Design review of the part shown in the three views and the two pictorial views. Dimensions are in mm from the part's minimum x, y and z. Give positions to 0.01 mm unless a question says otherwise; leave off trailing zeros. Order: outer loops, then holes, each group sorted by start corner. A loop starts at its lowest first (then second) coordinate and runs counter-clockwise, first axis right, second up.
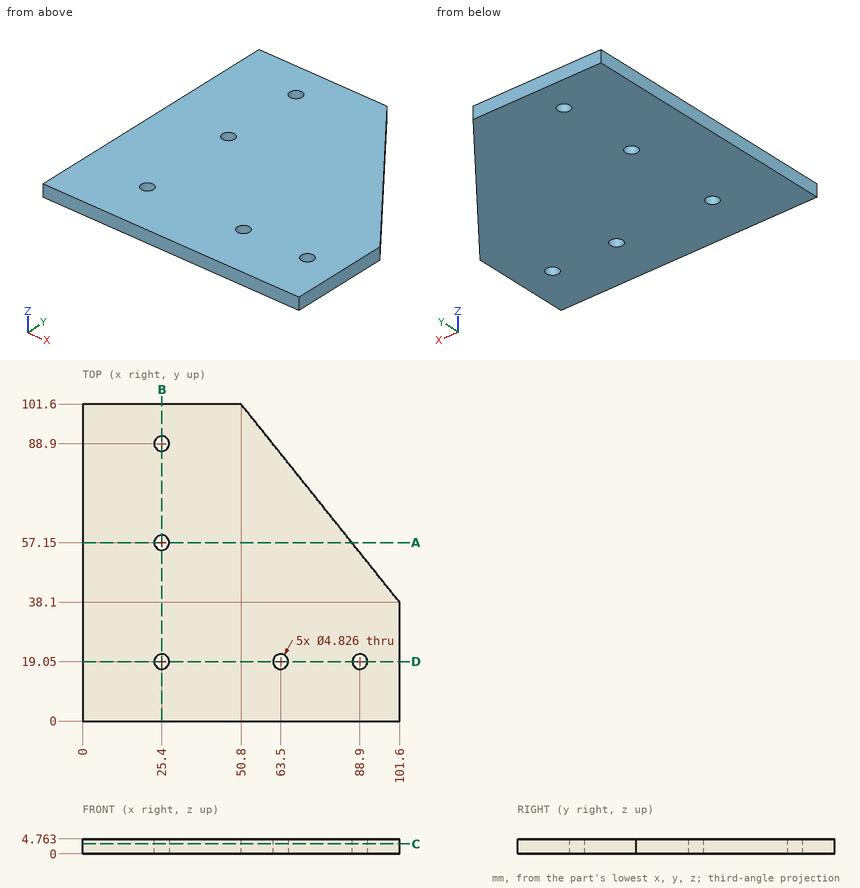
1) We need section D-D on y = 19.05. Give the boundary of the cut face in (x, z), then the cut area to 3 significant figures.
Answer sheet:
outline: (0, 0) - (22.99, 0) - (22.99, 4.76) - (0, 4.76) - close; (27.81, 0) - (61.09, 0) - (61.09, 4.76) - (27.81, 4.76) - close; (65.91, 0) - (86.49, 0) - (86.49, 4.76) - (65.91, 4.76) - close; (91.31, 0) - (101.6, 0) - (101.6, 4.76) - (91.31, 4.76) - close
area: 415 mm2
2) We need section B-B on x = 25.4. Give the boundary of the cut face in (y, z), then the cut area to 3 significant figures.
Answer sheet:
outline: (0, 0) - (16.64, 0) - (16.64, 4.76) - (0, 4.76) - close; (21.46, 0) - (54.74, 0) - (54.74, 4.76) - (21.46, 4.76) - close; (59.56, 0) - (86.49, 0) - (86.49, 4.76) - (59.56, 4.76) - close; (91.31, 0) - (101.6, 0) - (101.6, 4.76) - (91.31, 4.76) - close
area: 415 mm2
3) We need section A-A on y = 57.15. Give the boundary of the cut face in (x, z), then the cut area to 3 significant figures.
Answer sheet:
outline: (0, 0) - (22.99, 0) - (22.99, 4.76) - (0, 4.76) - close; (27.81, 0) - (86.36, 0) - (86.36, 4.76) - (27.81, 4.76) - close
area: 388 mm2
4) Clearance check with a flat-ended pin moving along its axis: pin 1 (3 mm diameter, centred on x = 25.4, y = 88.9, fed in from -Z). State where the tip first meets the part, or that it passes through.
Answer sheet:
pin 1: passes through
5) We need section C-C on z = 3.2. Count the separate pieces of the cut face and the enclosed holes in it, then the cut area to 3 significant figures.
Answer sheet:
separate pieces: 1
enclosed holes: 5
area: 8,620 mm2
6) To check wall thickness, follow line 1 (Y direction, x = 25.4, z = 1.2); line 2 (X direction, y = 19.05, z = 2.9); line 3 (X direction, y = 20, z = 0.9). State the ranges of each line that lie inside material, in increasing order.
Answer sheet:
line 1: y = 0 to 16.64, 21.46 to 54.74, 59.56 to 86.49, 91.31 to 101.6
line 2: x = 0 to 22.99, 27.81 to 61.09, 65.91 to 86.49, 91.31 to 101.6
line 3: x = 0 to 23.18, 27.62 to 61.28, 65.72 to 86.68, 91.12 to 101.6
